Input: part model. Units: mm. Frame: model coordinates. Face numbers are marked on the shaded views. A direction names the side the tool comes from. Coordinates: 2 decimals unless noted, no trailing zeros. Loops run counter-clockwise (first coordinate to the right, second up) from the corner with the lowest first, then second, coordinate; pieces in that order, holes last.
Item 1: Section B-B on x = -26.5. Return loops of the section in (y, z), and give its area (3 significant figures).
Item 2: Section C-C on z = -20.5. Return loops of the section in (x, y), and give its area (3 significant figures).
Item 3: Contact query for flat-ended pins moving along their axis: P1, Ø3.5, axis at x = 0, z = 20.5, coming from the +Y side; P2, Ø1, axis at x = -4.5, y = 1.5, coming from the +Z side; P3, Ø1, axis at x = 14, y = 5.5, coming from the -Z side. Output: stop coordinate, or through.
Item 4: Pull-direction query (X, two-part tool) for the marked faces 3, 4 and 5; classes: released by +X, released by -X, zero draft, split by the parting line, or undercut.
Item 5: Reachability of the marked faces 1 and 2 from +Z, -Z, +X, -X, +Y, -Y: full face, straight path, thin tool, end or side. Return the list, or none.
Item 6: Section D-D on y = 4.25. Give the number of separate pieces and of enclosed holes in the cut face, and give its area (3 significant figures).
Item 7: Ray query, line 1 along X through (y, z) = (5.1, 0); line 2 along Z through (x, y) = (8.5, 4.45); line 3 along X through (y, z) = (1.4, 23.5). Return the intervals inside material, ascending.
Item 8: Section A-A on z = -8.5. Return loops of the section in (x, y), and give its area (3 significant figures).
```python
from build123d import *

# Parameters (mm, degrees)
SKETCH1_R           = 35
SKETCH1_R_2         = 3
SKETCH1_R_3         = 1.5
SKETCH1_R_4         = 4.75
SKETCH1_R_5         = 3.25
BOSS_EXTRUDE2_DEPTH = 6
CUT_EXTRUDE3_START  = 6
SKETCH1_6_R         = 3
CUT_EXTRUDE3_DEPTH  = 3
SKETCH1_7_R         = 3
SKETCH1_7_R_2       = 1.5
BOSS_EXTRUDE3_DEPTH = 3


with BuildPart() as part:
    # Sketch1 → Boss-Extrude2 (new body)
    with BuildSketch(Plane(origin=(0, 0, 0), x_dir=(1, 0, 0), z_dir=(0, 1, 0))):
        Circle(SKETCH1_R)
        with BuildLine():
            Line((-29.580398915, -5), (-22.449944321, -5))
            ThreePointArc((-22.449944321, -5), (-21.249229248, -8.801718944), (-19.410041772, -12.33897396))
            Line((-19.410041772, -12.33897396), (-24.452034569, -17.380966757))
            ThreePointArc((-24.452034569, -17.380966757), (-27.716385975, -11.480502971), (-29.580398915, -5))
        make_face(mode=Mode.SUBTRACT)
        with BuildLine():
            Line((-17.380966757, -24.452034569), (-12.33897396, -19.410041772))
            ThreePointArc((-12.33897396, -19.410041772), (-8.801718944, -21.249229248), (-5, -22.449944321))
            Line((-5, -22.449944321), (-5, -29.580398915))
            ThreePointArc((-5, -29.580398915), (-11.480502971, -27.716385975), (-17.380966757, -24.452034569))
        make_face(mode=Mode.SUBTRACT)
        with BuildLine():
            Line((5, -29.580398915), (5, -22.449944321))
            ThreePointArc((5, -22.449944321), (8.801718944, -21.249229248), (12.33897396, -19.410041772))
            Line((12.33897396, -19.410041772), (17.380966757, -24.452034569))
            ThreePointArc((17.380966757, -24.452034569), (11.480502971, -27.716385975), (5, -29.580398915))
        make_face(mode=Mode.SUBTRACT)
        with BuildLine():
            Line((24.452034569, -17.380966757), (19.410041772, -12.33897396))
            ThreePointArc((19.410041772, -12.33897396), (21.249229248, -8.801718944), (22.449944321, -5))
            Line((22.449944321, -5), (29.580398915, -5))
            ThreePointArc((29.580398915, -5), (27.716385975, -11.480502971), (24.452034569, -17.380966757))
        make_face(mode=Mode.SUBTRACT)
        with BuildLine():
            Line((29.580398915, 5), (22.449944321, 5))
            ThreePointArc((22.449944321, 5), (21.249229248, 8.801718944), (19.410041772, 12.33897396))
            Line((19.410041772, 12.33897396), (24.452034569, 17.380966757))
            ThreePointArc((24.452034569, 17.380966757), (27.716385975, 11.480502971), (29.580398915, 5))
        make_face(mode=Mode.SUBTRACT)
        with BuildLine():
            Line((17.380966757, 24.452034569), (12.33897396, 19.410041772))
            ThreePointArc((12.33897396, 19.410041772), (8.801718944, 21.249229248), (5, 22.449944321))
            Line((5, 22.449944321), (5, 29.580398915))
            ThreePointArc((5, 29.580398915), (11.480502971, 27.716385975), (17.380966757, 24.452034569))
        make_face(mode=Mode.SUBTRACT)
        with BuildLine():
            Line((-5, 29.580398915), (-5, 22.449944321))
            ThreePointArc((-5, 22.449944321), (-8.801718944, 21.249229248), (-12.33897396, 19.410041772))
            Line((-12.33897396, 19.410041772), (-17.380966757, 24.452034569))
            ThreePointArc((-17.380966757, 24.452034569), (-11.480502971, 27.716385975), (-5, 29.580398915))
        make_face(mode=Mode.SUBTRACT)
        with BuildLine():
            Line((-24.452034569, 17.380966757), (-19.410041772, 12.33897396))
            ThreePointArc((-19.410041772, 12.33897396), (-21.249229248, 8.801718944), (-22.449944321, 5))
            Line((-22.449944321, 5), (-29.580398915, 5))
            ThreePointArc((-29.580398915, 5), (-27.716385975, 11.480502971), (-24.452034569, 17.380966757))
        make_face(mode=Mode.SUBTRACT)
        with Locations((0, -20.5)):
            Circle(SKETCH1_R_2, mode=Mode.SUBTRACT)
        with Locations((-20.5, 0)):
            Circle(SKETCH1_R_3, mode=Mode.SUBTRACT)
        with BuildLine():
            Line((-12.951558266, -1.121221875), (-17.932926829, -1.552461058))
            ThreePointArc((-17.932926829, -1.552461058), (-17.5, 0), (-17.932926829, 1.552461058))
            Line((-17.932926829, 1.552461058), (-12.951558266, 1.121221875))
            ThreePointArc((-12.951558266, 1.121221875), (-13, 0), (-12.951558266, -1.121221875))
        make_face(mode=Mode.SUBTRACT)
        with Locations((-4.75, 0)):
            Circle(SKETCH1_R_4, mode=Mode.SUBTRACT)
        with Locations((4.75, 0)):
            Circle(SKETCH1_R_5, mode=Mode.SUBTRACT)
        with BuildLine():
            ThreePointArc((17.932926829, 1.552461058), (17.5, 0), (17.932926829, -1.552461058))
            Line((17.932926829, -1.552461058), (12.951558266, -1.121221875))
            ThreePointArc((12.951558266, -1.121221875), (13, 0), (12.951558266, 1.121221875))
            Line((12.951558266, 1.121221875), (17.932926829, 1.552461058))
        make_face(mode=Mode.SUBTRACT)
        with Locations((20.5, 0)):
            Circle(SKETCH1_R_3, mode=Mode.SUBTRACT)
        with Locations((0, 20.5)):
            Circle(SKETCH1_R_2, mode=Mode.SUBTRACT)
    extrude(amount=BOSS_EXTRUDE2_DEPTH)

    # Sketch1<6> → Cut-Extrude3 (cut)
    with BuildSketch(Plane(origin=(0, 0, 0), x_dir=(1, 0, 0), z_dir=(0, 1, 0)).offset(CUT_EXTRUDE3_START)):
        with Locations((20.5, 0)):
            Circle(SKETCH1_6_R)
        with Locations((-20.5, 0)):
            Circle(SKETCH1_6_R)
    extrude(amount=-CUT_EXTRUDE3_DEPTH, mode=Mode.SUBTRACT)

    # Sketch1<7> → Boss-Extrude3 (add)
    with BuildSketch(Plane(origin=(0, 0, 0), x_dir=(1, 0, 0), z_dir=(0, 1, 0))):
        with Locations((0, 20.5)):
            Circle(SKETCH1_7_R)
        with Locations((0, 20.5)):
            Circle(SKETCH1_7_R_2, mode=Mode.SUBTRACT)
        with Locations((0, -20.5)):
            Circle(SKETCH1_7_R)
        with Locations((0, -20.5)):
            Circle(SKETCH1_7_R_2, mode=Mode.SUBTRACT)
    extrude(amount=BOSS_EXTRUDE3_DEPTH)


solid = part.part
```
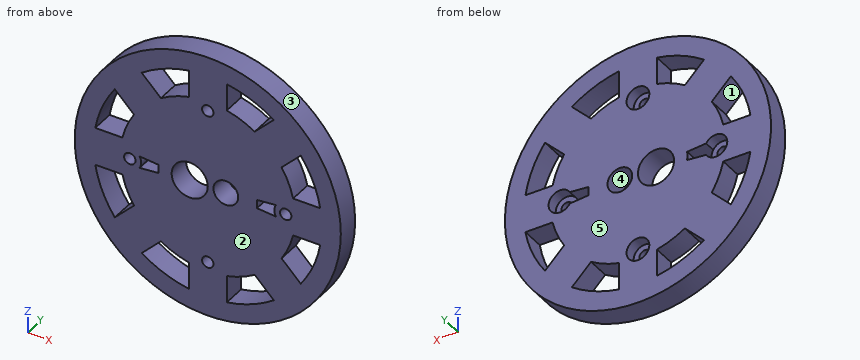
Results found:
1. outline: (0, -22.86) - (6, -22.86) - (6, -14.06) - (0, -14.06) - close; (0, -5) - (6, -5) - (6, 5) - (0, 5) - close; (0, 14.06) - (6, 14.06) - (6, 22.86) - (0, 22.86) - close
1. area: 166 mm2
2. outline: (-28.37, 0) - (-13.43, 0) - (-13.43, 6) - (-28.37, 6) - close; (-10.43, 0) - (-1.5, 0) - (-1.5, 3) - (-3, 3) - (-3, 6) - (-10.43, 6) - close; (1.5, 0) - (10.43, 0) - (10.43, 6) - (3, 6) - (3, 3) - (1.5, 3) - close; (13.43, 0) - (28.37, 0) - (28.37, 6) - (13.43, 6) - close
2. area: 277 mm2
3. P1: stops at y = 3
3. P2: stops at z = 34.77
3. P3: stops at z = -32.29
4. face 3: split by the parting line
4. face 4: undercut
4. face 5: zero draft
5. face 1: +Y, -Y
5. face 2: +Z, -Z, +X, -X, -Y
6. separate pieces: 1
6. enclosed holes: 14
6. area: 3,000 mm2
7. line 1: x = -35 to -23.5, -13 to -9.5, 0 to 1.5, 8 to 13, 23.5 to 35
7. line 2: z = -33.95 to -28.77, -21.37 to 21.37, 28.77 to 33.95
7. line 3: x = -25.94 to -16.43, -5 to 5, 16.43 to 25.94
8. outline: (-33.95, 0) - (-28.77, 0) - (-28.77, 6) - (-33.95, 6) - close; (-21.37, 0) - (21.37, 0) - (21.37, 6) - (-21.37, 6) - close; (28.77, 0) - (33.95, 0) - (33.95, 6) - (28.77, 6) - close
8. area: 319 mm2
